Model file for the job. Use its own axes, mm. A direction names the side the tool comes from. Coordinates: 2 decimals unless noted, no trailing zeros. Order: outer loops, then holes, each group sorted by start corner. A loop starts at its lowest first (then second) coordinate and runs counter-clockwise, first axis right, second up. Notation, with made-up numbers: (-18, 78.25) - (19, 78.25) arc R3 cw to (19, 83.25) - close; hole circle Ø3 at (53, 20). An arc over 180 degrees is marked (long way). Put each result on its own line as item: value. Start each with the question number.
```python
from build123d import *

# Parameters (mm, degrees)
SKETCH1_R           = 40
BOSS_EXTRUDE1_DEPTH = 40


with BuildPart() as part:
    # Sketch1 → Boss-Extrude1 (new, symmetric)
    with BuildSketch(Plane(origin=(0, 0, 0), x_dir=(0, 0, -1), z_dir=(1, 0, 0))):
        with BuildLine():
            Line((-53, -29.1), (-42.369210519, -29.1))
            ThreePointArc((-42.369210519, -29.1), (0, -51.4), (42.369210519, -29.1))
            Line((42.369210519, -29.1), (53, -29.1))
            Line((53, -29.1), (53, 39))
            Line((53, 39), (74, 39))
            Line((74, 39), (74, 53))
            Line((74, 53), (-74, 53))
            Line((-74, 53), (-74, 39))
            Line((-74, 39), (-53, 39))
            Line((-53, 39), (-53, -29.1))
        make_face()
        Circle(SKETCH1_R, mode=Mode.SUBTRACT)
    extrude(amount=BOSS_EXTRUDE1_DEPTH, both=True)


solid = part.part
```
Item 1: Flat gauge pins, fed straight in: pin 1 Ø6 at (x, y) = (16.5, 22.5) entering from -Z; pin 2 Ø10.5 at (x, z) = (-18, -65) entering from -Y; pin 3 Ø11.5 at (x, z) = (-14, -46.5) entering from -Y. Where does each tip first touch, or does it go through?
Item 2: Wall check: line 1 along Y through (x, z) = (8, 0); line 2 along Y through (x, z) = (12, 64.5); line 3 along Z through (x, y) = (34.5, 4). Give the ranges that are in metal, low to high.
Item 3: Slice it at A-A, the plane z = 0. Give the cut face in (x, y).
Item 4: Slice it at D-D, the plane z = -59.5. Give the cut face in (x, y).
Item 5: 3-axis set-ups, long thin cutter, end or side, ignore diameter. For faces 1 (the face through (1, -29.1, -48)), 2 (the face through (1, 5, 53)), 3 (the face through (1, 53, -1)): which of +Z, -Z, +X, -X, +Y, -Y reach the whole face in a straight line?
Item 6: Slice it at B-B, the plane x = -11. Give the cut face in (y, z).
Item 7: Slice it at C-C, the plane y = 0. Give the cut face in (x, z).
Item 8: Pull direction Y, two halves, no side cores. Call faces 4 (the face through (0.56, -51.395, 0.697)), 5 (the face through (-0.56, -39.05, 8.67)), 6 (the face through (40, 36.3, 17.5)): pulls with the +Y half, pulls with the -Y half, needs draft (parallel to the pull), parting line crosses it, or undercut.
Here are the results:
1. pin 1: stops at z = -53
1. pin 2: stops at y = 39
1. pin 3: stops at y = -31.33
2. line 1: y = -51.4 to -40, 40 to 53
2. line 2: y = 39 to 53
2. line 3: z = -53 to -39.8, 39.8 to 53
3. outline: (-40, -51.4) - (40, -51.4) - (40, -40) - (-40, -40) - close; (-40, 40) - (40, 40) - (40, 53) - (-40, 53) - close
4. outline: (-40, 39) - (40, 39) - (40, 53) - (-40, 53) - close
5. face 1: -Z, +X, -X, -Y
5. face 2: +Z, +X, -X, -Y
5. face 3: +Z, -Z, +X, -X, +Y
6. outline: (-29.1, -53) - (39, -53) - (39, -74) - (53, -74) - (53, 74) - (39, 74) - (39, 53) - (-29.1, 53) - (-29.1, 42.37) arc R51.4 ccw to (-29.1, -42.37) - close; hole circle Ø80 at (0, 0)
7. outline: (-40, -53) - (40, -53) - (40, -40) - (-40, -40) - close; (-40, 40) - (40, 40) - (40, 53) - (-40, 53) - close
8. face 4: pulls with the -Y half
8. face 5: undercut
8. face 6: needs draft
